from build123d import *

# Parameters (mm, degrees)
SKETCH1_W         = 258
SKETCH1_H         = 293
MAIN_BASE_DEPTH   = 3.175
ALIGNMENT_HOLES_D = 12


with BuildPart() as part:
    # Sketch1 → Main Base (new, symmetric)
    with BuildSketch(Plane(origin=(0, 0, 0), x_dir=(1, 0, 0), z_dir=(0, 1, 0))):
        Rectangle(SKETCH1_W, SKETCH1_H)
    extrude(amount=MAIN_BASE_DEPTH, both=True)

    # Alignment Holes (through all)
    with Locations(Plane(origin=(0, 3.175, 0), x_dir=(1, 0, 0), z_dir=(0, 1, 0))):
        with Locations((-107.5, 0), (-43, -37.239092363), (-43, 37.239092363), (86, 37.239092363), (21.5, 0), (86, -37.239092363), (-107.5, 74.478184725), (-43, 111.717277088), (21.5, 74.478184725), (86, 111.717277088), (-107.5, -74.478184725), (-43, -111.717277088), (21.5, -74.478184725), (86, -111.717277088)):
            Hole(ALIGNMENT_HOLES_D / 2)


solid = part.part
Can you work these out from the model? Positions are in its coordinate system, mm. Round coordinates to 2 decimals unless told otherwise and drop trailing zeros. Write each loop counter-clockwise with the first axis right and the second up, starting at its lowest first coordinate (ties: lowest second). Pieces come first, ordered by that corner, then holes. Notation, with made-up numbers: M 6.25,44 L 59.25,44 A16 cw 59.25,53 Z; hole C 18.5,10.5 d1. An arc over 180 degrees is marked long. Use a Markdown table: item, result.
Item 1: I want a section at C-C (x = 86). List the corners of the cut face in (y, z) for me (3 decimals).
Found:
| item | result |
|---|---|
| outline | M -3.175,-146.5 L 3.175,-146.5 L 3.175,-117.717 L -3.175,-117.717 Z; M -3.175,-105.717 L 3.175,-105.717 L 3.175,-43.239 L -3.175,-43.239 Z; M -3.175,-31.239 L 3.175,-31.239 L 3.175,31.239 L -3.175,31.239 Z; M -3.175,43.239 L 3.175,43.239 L 3.175,105.717 L -3.175,105.717 Z; M -3.175,117.717 L 3.175,117.717 L 3.175,146.5 L -3.175,146.5 Z |
Item 2: We'd pull the mould along Z, two halves only. Please class faces 1 (the face through (-2, 0, 146.5)), 2 (the face through (-101.506, -0.044, 74.214)), 3 (the face through (87.301, -0.044, 117.575)), 4 (the face through (-2, -3.175, -2)): released by +Z, released by -Z, zero draft, split by the parting line, or undercut.
Found:
| item | result |
|---|---|
| face 1 | released by +Z |
| face 2 | undercut |
| face 3 | undercut |
| face 4 | zero draft |
Item 3: If I drill on line 1 along Z through (x, y) = (-43, -1.5); line 2 along Z through (x, y) = (21.5, 1.5); line 3 along X through (y, z) = (0, 1), over which ranges is the centre line in solid material (lowest first)? Write a range as [from, to].
Found:
| item | result |
|---|---|
| line 1 | z = [-146.5, -117.72], [-105.72, -43.24], [-31.24, 31.24], [43.24, 105.72], [117.72, 146.5] |
| line 2 | z = [-146.5, -80.48], [-68.48, -6], [6, 68.48], [80.48, 146.5] |
| line 3 | x = [-129, -113.42], [-101.58, 15.58], [27.42, 129] |
Item 4: I want a section at B-B (x = -107.5). List the corners of the cut face in (y, z) for me (3 decimals), and give its area (3 significant figures).
Found:
| item | result |
|---|---|
| outline | M -3.175,-146.5 L 3.175,-146.5 L 3.175,-80.478 L -3.175,-80.478 Z; M -3.175,-68.478 L 3.175,-68.478 L 3.175,-6 L -3.175,-6 Z; M -3.175,6 L 3.175,6 L 3.175,68.478 L -3.175,68.478 Z; M -3.175,80.478 L 3.175,80.478 L 3.175,146.5 L -3.175,146.5 Z |
| area | 1,630 mm2 |
Item 5: For pin 1 Ø19 at (x, z) = (-43, 37.24) entering from -Y (3 decimals), with a flat end and sliding along its axis, tell me the tip position at first contact or that it passes through.
Found:
| item | result |
|---|---|
| pin 1 | stops at y = -3.175 |
Item 6: I want a section at A-A (z = 0). List the corners of the cut face in (x, y) for me (3 decimals), and give its area (3 significant figures).
Found:
| item | result |
|---|---|
| outline | M -129,-3.175 L -113.5,-3.175 L -113.5,3.175 L -129,3.175 Z; M -101.5,-3.175 L 15.5,-3.175 L 15.5,3.175 L -101.5,3.175 Z; M 27.5,-3.175 L 129,-3.175 L 129,3.175 L 27.5,3.175 Z |
| area | 1,490 mm2 |
Item 7: I want a section at D-D (y = -0.25). State how many separate pieces and enclosed holes the cut face has, and give its area (3 significant figures).
Found:
| item | result |
|---|---|
| separate pieces | 1 |
| enclosed holes | 14 |
| area | 74,000 mm2 |
